Could you check a few things on this model? Use its own coordinates, in mm. Face numbers are marked on the shaded views. A direction names the side the tool comes from. Coordinates: 2 decimals unless noted, no trailing zeros. Order: outer loops, then holes, each group sorted by start corner. A loop starts at its lowest first (then second) coordinate and runs counter-clockwise, first axis right, second up. Notation, with made-up numbers: (47, -39) - (92, -39) arc R23 ccw to (92, -21) - close; hole circle Ø3 at (72.5, -34). An arc over 180 degrees is marked (long way). Answer as CSV lines item,"result". Start each with the question number.
1. For the marked faces 1 and 2, which set-ups out of +Z, -Z, +X, -X, +Y, -Y let a thin tool reach every point of the face, with its end or its side?
2. I want a section at A-A, the plane x = 0. List the corners of the cut face in (y, z) for me.
3. For pin 1 (1.5 mm diameter, centred on y = 15, z = 1, fed in from -X); pin 2 (1.5 mm diameter, centred on x = 44, z = 2, fed in from -Y); pin 3 (0.5 mm diameter, centred on y = -11, z = 4.5, fed in from -X); pin 4 (12 mm diameter, centred on x = 7, y = 12, fed in from -Z), each with a flat end and sliding along its axis, tell me the tip position at first contact or that it passes through.
4. I need wall thicknesses on probe 1 along Y at (x, z) = (56, 1.5); probe 2 along X at (y, z) = (-6, 3); probe 3 along X at (y, z) = (-8, 4). Which ranges of each line are inside material? Lowest first, please.
5. I want a section at D-D, the plane y = -40. List the corners of the cut face in (x, z) for me, and give its area (3 significant figures).
6. I want a section at C-C, the plane x = -51. List the corners of the cut face in (y, z) for me.
7. I want a section at B-B, the plane z = 5.25. List the corners of the cut face in (x, y) for me.
8. Thinking about a two-plate mould opening in X: for the marked faces 3, 4 and 5, which applies, released by +X, released by -X, zero draft, split by the parting line, or undercut?
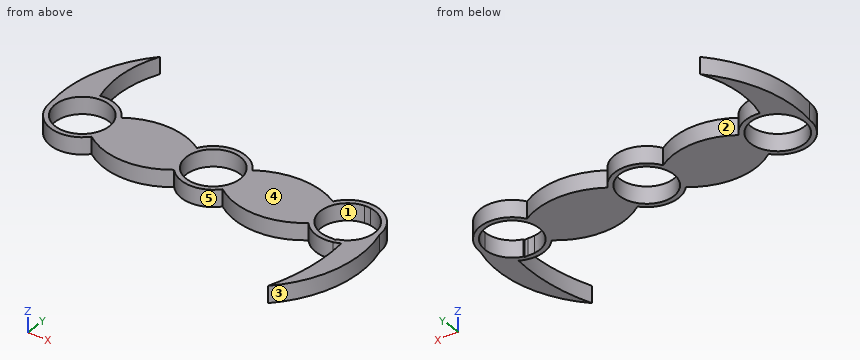
from build123d import *

# Parameters (mm, degrees)
F0_R     = 11.2
F1_DEPTH = 7


with BuildPart() as f1:
    # F0 (on Top) → F1 (new body)
    with BuildSketch(Plane.XY):
        with BuildLine():
            ThreePointArc((44.39689, 7.089599), (27.857047, 11.450683), (11.478691, 6.517641))
            ThreePointArc((11.478691, 6.517641), (0, 13.2), (-11.478691, 6.517641))
            ThreePointArc((-11.478691, 6.517641), (-27.06632, 11.210689), (-42.653949, 6.517641))
            ThreePointArc((-42.653949, 6.517641), (-48.387541, 11.884184), (-56.154664, 13.04421))
            ThreePointArc((-56.154664, 13.04421), (-64.155881, 8.589217), (-67.33264, 0))
            ThreePointArc((-67.33264, 0), (-58.723405, -12.37598), (-44.12584, -8.608365))
            ThreePointArc((-44.12584, -8.608365), (-27.06632, -14.299813), (-10.0068, -8.608365))
            ThreePointArc((-10.0068, -8.608365), (0, -13.2), (10.0068, -8.608365))
            ThreePointArc((10.0068, -8.608365), (27.689109, -14.41312), (45.267037, -8.299554))
            ThreePointArc((45.267037, -8.299554), (51.281831, -12.497242), (58.608726, -12.836282))
            ThreePointArc((58.608726, -12.836282), (60.045688, -12.404085), (61.424313, -11.811593))
            ThreePointArc((61.424313, -11.811593), (66.75697, -6.944556), (68.731412, 0))
            ThreePointArc((68.731412, 0), (59.223587, 12.673115), (44.39689, 7.089599))
        make_face()
        with Locations((-54.13264, 0)):
            Circle(F0_R, mode=Mode.SUBTRACT)
        Circle(F0_R, mode=Mode.SUBTRACT)
        with BuildLine():
            Line((58.608726, -10.768943), (58.608726, -11.2))
            ThreePointArc((58.608726, -11.2), (57.837567, -11.17342), (57.070069, -11.093806))
            ThreePointArc((57.070069, -11.093806), (55.742724, -11.198006), (54.412393, -11.143958))
            ThreePointArc((54.412393, -11.143958), (44.331412, 0), (54.412393, 11.143958))
            ThreePointArc((54.412393, 11.143958), (55.742724, 11.198006), (57.070069, 11.093806))
            ThreePointArc((57.070069, 11.093806), (63.977505, 7.35551), (66.731412, 0))
            ThreePointArc((66.731412, 0), (64.473054, -6.744408), (58.608726, -10.768943))
        make_face(mode=Mode.SUBTRACT)
        with BuildLine():
            ThreePointArc((-67.33264, 0), (-64.155881, 8.589217), (-56.154664, 13.04421))
            ThreePointArc((-56.154664, 13.04421), (-57.711729, 28.652134), (-53.573128, 43.781698))
            ThreePointArc((-53.573128, 43.781698), (-65.554278, 23.494092), (-67.33264, 0))
        make_face()
        with BuildLine():
            ThreePointArc((56.362603, -46.893224), (69.078735, -25.169456), (68.731412, 0))
            ThreePointArc((68.731412, 0), (66.75697, -6.944556), (61.424313, -11.811593))
            ThreePointArc((61.424313, -11.811593), (60.986371, -29.654382), (56.362603, -46.893224))
        make_face()
    extrude(amount=F1_DEPTH)


solid = f1.part
Solved:
1,face 1,"+Z, -Z"
1,face 2,"+Z, -Z, +Y"
2,outline,"(-13.2, 0) - (-11.2, 0) - (-11.2, 7) - (-13.2, 7) - close; (11.2, 0) - (13.2, 0) - (13.2, 7) - (11.2, 7) - close"
3,pin 1,"stops at x = -67.56"
3,pin 2,"stops at y = -9.73"
3,pin 3,"stops at x = -61.79"
3,pin 4,"stops at z = 0"
4,probe 1,"y = -13.19 to -11.19, 11.19 to 13.19"
4,probe 2,"x = -65.89 to -63.59, -44.68 to -9.46, 9.46 to 46.07, 64.99 to 70.07"
4,probe 3,"x = -64.63 to -61.97, -46.29 to -7.84, 7.84 to 47.69, 63.37 to 70.34"
5,outline,"(58.74, 0) - (62.22, 0) - (62.22, 7) - (58.74, 7) - close"
5,area,"24.4 mm2"
6,outline,"(-12.82, 0) - (-10.75, 0) - (-10.75, 7) - (-12.82, 7) - close; (10.75, 0) - (12.82, 0) - (12.82, 7) - (10.75, 7) - close"
7,outline,"(-67.33, 0) arc R13.2 ccw to (-44.13, -8.61) arc R28.41 ccw to (-10.01, -8.61) arc R13.2 ccw to (10.01, -8.61) arc R29.06 ccw to (45.27, -8.3) arc R13.2 ccw to (58.61, -12.84) arc R13.2 ccw to (61.42, -11.81) arc R75.32 cw to (56.36, -46.89) arc R46.9 ccw to (68.73, 0) arc R13.2 ccw to (44.4, 7.09) arc R31.48 ccw to (11.48, 6.52) arc R13.2 ccw to (-11.48, 6.52) arc R28.23 ccw to (-42.65, 6.52) arc R13.2 ccw to (-56.15, 13.04) arc R43.04 cw to (-53.57, 43.78) arc R51.91 ccw to start; hole circle Ø22.4 at (-54.13, 0); hole circle Ø22.4 at (0, 0); hole (54.41, -11.14) arc R11.2 ccw to (57.07, -11.09) arc R11.2 ccw to (58.61, -11.2) - (58.61, -10.77) arc R11.2 ccw to (66.73, 0) arc R11.2 ccw to (57.07, 11.09) arc R11.2 ccw to (54.41, 11.14) arc R11.2 ccw to start"
8,face 3,"released by +X"
8,face 4,"zero draft"
8,face 5,"undercut"
